from build123d import *

# Parameters (mm, degrees)
BOX002_W          = 6.4
BOX002_H          = 11.8
BOX002_DEPTH      = 1.6
CYLINDER002_R     = 1.35
CYLINDER002_DEPTH = 10
CYLINDER001_R     = 1.35
CYLINDER001_DEPTH = 10
CYLINDER_R        = 1.35
CYLINDER_DEPTH    = 10
BOX_W             = 1.6
BOX_H             = 22
BOX_DEPTH         = 14.5
BOX001_W          = 6.4
BOX001_H          = 11.8
BOX001_DEPTH      = 1.6
CYLINDER003_R     = 1.35
CYLINDER003_DEPTH = 10
BOX003_W          = 6.4
BOX003_H          = 11.8
BOX003_DEPTH      = 1.6
EXTRUDE_DEPTH     = 1.6


with BuildPart() as cube002:
    # Box002 → Box002 (new body)
    with BuildSketch(Plane(origin=(1.6, 0, 0), x_dir=(1, 0, 0), z_dir=(0, 0, 1))):
        with Locations((3.2, 5.9)):
            Rectangle(BOX002_W, BOX002_H)
    extrude(amount=BOX002_DEPTH)


with BuildPart() as cylinder002:
    # Cylinder002 → Cylinder002 (new body)
    with BuildSketch(Plane(origin=(4, 5.5, 0), x_dir=(1, 0, 0), z_dir=(0, 0, 1))):
        Circle(CYLINDER002_R)
    extrude(amount=CYLINDER002_DEPTH)


with BuildPart() as cylinder001:
    # Cylinder001 → Cylinder001 (new body)
    with BuildSketch(Plane(origin=(0, 16.5, 9), x_dir=(0, 0, -1), z_dir=(1, 0, 0))):
        Circle(CYLINDER001_R)
    extrude(amount=CYLINDER001_DEPTH)


with BuildPart() as cylinder:
    # Cylinder → Cylinder (new body)
    with BuildSketch(Plane(origin=(0, 5.5, 9), x_dir=(0, 0, -1), z_dir=(1, 0, 0))):
        Circle(CYLINDER_R)
    extrude(amount=CYLINDER_DEPTH)


with BuildPart() as cut001:
    # Box → Box (new body)
    with BuildSketch(Plane.XY):
        with Locations((0.8, 11)):
            Rectangle(BOX_W, BOX_H)
    extrude(amount=BOX_DEPTH)

    # Cut: cut Cylinder
    add(cylinder.part, mode=Mode.SUBTRACT)

    # Cut001: cut Cylinder001
    add(cylinder001.part, mode=Mode.SUBTRACT)


with BuildPart() as cut003:
    # Box001 → Box001 (new body)
    with BuildSketch(Plane(origin=(1.6, 0, 0), x_dir=(1, 0, 0), z_dir=(0, 0, 1))):
        with Locations((3.2, 5.9)):
            Rectangle(BOX001_W, BOX001_H)
    extrude(amount=BOX001_DEPTH)

    # Connect: union Cut001
    add(cut001.part)

    # Cut002: cut Cylinder002
    add(cylinder002.part, mode=Mode.SUBTRACT)

    # Cut003: cut Cube002
    add(cube002.part, mode=Mode.SUBTRACT)


with BuildPart() as cylinder003:
    # Cylinder003 → Cylinder003 (new body)
    with BuildSketch(Plane(origin=(4, 16.5, 0), x_dir=(1, 0, 0), z_dir=(0, 0, 1))):
        Circle(CYLINDER003_R)
    extrude(amount=CYLINDER003_DEPTH)


with BuildPart() as cut004:
    # Box003 → Box003 (new body)
    with BuildSketch(Plane(origin=(1.6, 10.2, 0), x_dir=(1, 0, 0), z_dir=(0, 0, 1))):
        with Locations((3.2, 5.9)):
            Rectangle(BOX003_W, BOX003_H)
    extrude(amount=BOX003_DEPTH)

    # Cut004: cut Cylinder003
    add(cylinder003.part, mode=Mode.SUBTRACT)


with BuildPart() as connect001:
    # Sketch → Extrude (new body)
    with BuildSketch(Plane.XZ):
        Polygon((1.593675, 14.483153), (1.593675, 1.60001), (7.999931, 1.60001), align=None)
    extrude(amount=EXTRUDE_DEPTH)


with BuildPart() as connect001_1:
    # Extrude placement: moved
    add(connect001.part.moved(Location((0, 11.8, 0))))

    # Connect001: union Cut003, Cut004
    add(cut003.part)
    add(cut004.part)


solid = connect001_1.part
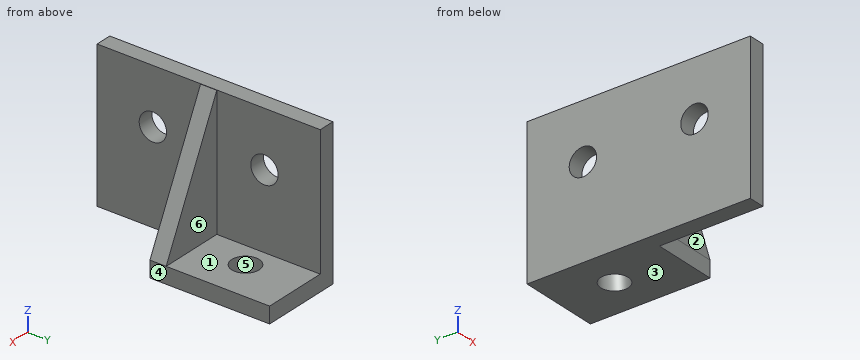
Build history of the part. All positions in model axes, mm. Face numbers are marked on the shaded views. A direction names the side the tool comes from. Round coordinates to 2 decimals unless told otherwise and drop trailing zeros. Write each loop counter-clockwise with the first axis right and the second up, starting at its lowest first coordinate (ties: lowest second). Pieces come first, ordered by that corner, then holes. Notation, with made-up numbers: M -30.5,14 L 17.5,14 A7 cw 17.5,27 Z; hole C 72.25,-10 d7. An arc over 180 degrees is marked long. Answer as a JSON object with one key per item and string values. Group by question number.
(1) Cut at A-A (y = 16.5). Give the cut face in (x, z), and give its area (3 significant figures).
(2) Cut at D-D (z = 9). Give the cut face in (x, y), and give its area (3 significant figures).
(3) Which spindle directions (+Z, -Z, +X, -X, +Y, -Y) get a long thin tool onto all of the face, cutting with end or side? Do the marked faces 1, 2 and 3. Say none if no direction does.
(4) Drill centre lines: L1, parallel to Y at x = 0.7, z = 9; L2, parallel to Z at x = 0.6, y = 16.5; L3, parallel to Y at x = 4, z = 1.3. Where is each one in solid material? Low to high.
(5) Flat gauge pins, fed straight in: pin 1 (1.5 mm diameter, centred on x = 3.5, z = 9, fed in from +Y); pin 2 (1.5 mm diameter, centred on x = 3, z = 10.5, fed in from -Y); pin 3 (3 mm diameter, centred on x = 5.5, y = 18, fed in from +Z). Where does each tip first touch, or does it go through?
(6) Mould opens along Y. For the marked faces 4, 5 and 6 say: pulls with the +Y half, pulls with the -Y half, needs draft (parallel to the pull), parting line crosses it, or undercut.
(7) Cut at C-C (x = 0.5). Give the cut face in (y, z).
(8) Cut at B-B (y = 5.5). Give the cut face in (x, z).
Responses:
{
 "1": {"outline": "M 0,0 L 2.65,0 L 2.65,1.6 L 1.6,1.6 L 1.6,7.65 L 0,7.65 Z; M 0,10.35 L 1.6,10.35 L 1.6,14.5 L 0,14.5 Z; M 5.35,0 L 8,0 L 8,1.6 L 5.35,1.6 Z", "area": "24.8 mm2"},
 "2": {"outline": "M 0,0 L 1.6,0 L 1.6,4.15 L 0,4.15 Z; M 0,6.85 L 1.6,6.85 L 1.6,10.2 L 4.32,10.2 L 4.32,11.8 L 1.6,11.8 L 1.6,15.15 L 0,15.15 Z; M 0,17.85 L 1.6,17.85 L 1.6,22 L 0,22 Z", "area": "30.9 mm2"},
 "3": {"face 1": "none", "face 2": "+Z, -Z, +X, -Y", "face 3": "-Z, +X, -X, +Y, -Y"},
 "4": {"L1": "y = 0 to 4.15, 6.85 to 15.15, 17.85 to 22", "L2": "z = 0 to 7.65, 10.35 to 14.5", "L3": "y = 10.2 to 15.15, 17.85 to 22"},
 "5": {"pin 1": "stops at y = 11.8", "pin 2": "stops at y = 10.2", "pin 3": "stops at z = 1.6"},
 "6": {"face 4": "needs draft", "face 5": "undercut", "face 6": "pulls with the +Y half"},
 "7": {"outline": "M 0,0 L 22,0 L 22,14.5 L 0,14.5 Z; hole C 5.5,9 d2.7; hole C 16.5,9 d2.7"},
 "8": {"outline": "M 0,0 L 1.6,0 L 1.6,7.65 L 0,7.65 Z; M 0,10.35 L 1.6,10.35 L 1.6,14.5 L 0,14.5 Z"}
}
